Source: CAD feature listing. Evaluate the final solid. Frame: model axes, mm. A direction names the side the tool comes from. Round coordinates to 2 decimals unless told otherwise and drop trailing zeros. Loops run counter-clockwise (first coordinate to the right, second up) from the corner with the lowest first, then second, coordinate; pieces in that order, holes last. Notation, with made-up numbers: (53.5, -29) - (67.5, -29) arc R13 ccw to (67.5, -19) - close; hole circle Ø8 at (-20, 43). An arc over 180 degrees is marked (long way). Write item = value, one per line. Start each with the question number.
from build123d import *

# Parameters (mm, degrees)
SALIENTE_EXTRUIR1_DEPTH = 1.5
CROQUIS2_W              = 2.9
CROQUIS2_H              = 14.8
CORTAR_EXTRUIR1_DEPTH   = 10


with BuildPart() as part:
    # Croquis1 → Saliente-Extruir1 (new, symmetric)
    with BuildSketch(Plane.XY):
        Polygon((497.855720503, 73.173038091), (497.855720503, 63.273038097), (494.855720505, 63.273038097), (494.855720505, 45.573091251), (491.106069484, 45.573091251), (491.106069484, 48.073510022), (488.105720509, 48.073510022), (488.105720509, 45.573091251), (487.13072051, 45.573091251), (487.13072051, 42.573091253), (488.105720509, 42.573091253), (488.105720509, 40.073091254), (491.106069484, 40.073091254), (491.106069484, 42.573091253), (494.855720505, 42.573091253), (494.855720505, 41.050309336), (494.855720505, 40.650309337), (494.855720505, 37.67310897), (497.855691931, 37.67310897), (497.855691931, 27.773108976), (494.855720505, 27.773108976), (494.855720505, 12.773108985), (479.205555648, 12.773108985), (468.814796849, 4.447241951), (463.814796852, 4.447241951), (465.108892077, 9.276871079), (462.2111146, 10.053328214), (464.799305049, 19.712586471), (467.697082526, 18.936129336), (471.203015891, 32.02045078), (474.824900651, 31.049969683), (474.177853039, 28.635155119), (477.075967602, 27.858607662), (477.723015214, 30.273422227), (478.664792894, 30.021073658), (479.441250029, 32.918851135), (478.499472349, 33.171199704), (479.146628347, 35.586418771), (476.248513785, 36.362966228), (475.601357786, 33.94774716), (471.979473025, 34.918228257), (476.379396799, 51.33896733), (480.001281419, 50.368486271), (479.354233806, 47.953671707), (482.252348369, 47.177124251), (482.899395981, 49.591938815), (483.841173662, 49.339590246), (484.617630796, 52.237367723), (483.675853116, 52.489716292), (484.323009115, 54.904935359), (481.424894552, 55.681482816), (480.777738553, 53.266263749), (477.155853934, 54.236744807), (480.661787289, 67.321066215), (477.764009811, 68.097523349), (480.352200261, 77.756781606), (483.249977738, 76.980324471), (484.855720511, 82.973038085), (494.855720505, 82.973038085), (494.855720505, 73.173038091), align=None)
    extrude(amount=SALIENTE_EXTRUIR1_DEPTH, both=True)

    # Croquis2 → Cortar-Extruir1 (cut)
    with BuildSketch(Plane.XY.offset(1.5)):
        with Locations((491.355720503, 62.973038085)):
            Rectangle(CROQUIS2_W, CROQUIS2_H)
    extrude(amount=-CORTAR_EXTRUIR1_DEPTH, mode=Mode.SUBTRACT)


solid = part.part
(1) Pin query (flat end, axial travel): P1, Ø1.5, axis at y = 78, z = -0.5, coming from the +X side; P2, Ø0.9, axis at x = 496.5, z = -0.5, coming from the -Y side; P3, Ø1.5, axis at x = 496.5, z = 0, coming from the +Y side. Return the tip coordinate at first contact, or that it passes through.
(2) Cut plane C-C (x = 470). Output: boundary loops of the cut face in (y, z), and give its area (3 significant figures).
(3) Cut plane A-A (x = 494). Output: boundary loops of the cut face in (y, z), and give its area (3 significant figures).
(4) Cut plane B-B (y = 25.5). Output: boundary loops of the cut face in (x, z), and give its area (3 significant figures).
(5) Mould query, pull axis X, two halves, no side actions, for faces 1 (the face through (496, 37.673, 0)), 2 (the face through (474.083, 8.668, 0.021)), 3 (the face through (479.048, 31.45, 0.021)). Classes: +X half, -X half, draft (parallel to the pull), parting line (faces both ways), or undercut.
(6) Access query for faces 4 (the face through (493, 42.573, 0)), 5 (the face through (480.78, 47.57, 0.02)), 6 (the face through (481.781, 77.374, 0.021)), 7 (the face through (473.816, 34.426, 0.021)). Directions: +Z, -Z, +X, -X, +Y, -Y. A direction counts if a zero-diameter tool reaches every point of the face in a straight line with its end or side. Return the directions, or none.
(7) Material intervals for line 1 along Y through (x, z) = (490.5, 0.7); line 2 along Y through (x, z) = (492.5, -0.65); line 3 along Y through (x, z) = (488, 0.95), sorted ascending. Write a range as from..to.
Solution:
q1.P1 = 494.86
q1.P2 = 27.77
q1.P3 = 73.17
q2.outline = (5.4, -1.5) - (27.53, -1.5) - (27.53, 1.5) - (5.4, 1.5) - close
q2.area = 66.4 mm^2
q3.outline = (12.77, -1.5) - (42.57, -1.5) - (42.57, 1.5) - (12.77, 1.5) - close; (45.57, -1.5) - (82.97, -1.5) - (82.97, 1.5) - (45.57, 1.5) - close
q3.area = 202 mm^2
q4.outline = (469.46, -1.5) - (494.86, -1.5) - (494.86, 1.5) - (469.46, 1.5) - close
q4.area = 76.2 mm^2
q5.face_1 = draft
q5.face_2 = +X half
q5.face_3 = undercut
q6.face_4 = +Z, -Z, +X
q6.face_5 = +Z, -Z
q6.face_6 = +Z, -Z, +Y
q6.face_7 = +Z, -Z, -X
q7.line_1 = 12.77..40.07, 48.07..55.57, 70.37..82.97
q7.line_2 = 12.77..42.57, 45.57..55.57, 70.37..82.97
q7.line_3 = 12.77..42.57, 45.57..82.97
